Model file for the job. Use its own axes, mm. Face numbers are marked on the shaded views. Coordinates: 2 decimals unless noted, no trailing zeros. Write each loop counter-clockwise with the first axis right and the second up, starting at its lowest first coordinate (ties: lowest second). Pieces come first, ordered by that corner, then holes.
Q1. Band-saw the part on B-B, the plane z = 43. Write the cut outline in (x, y).
Q2. Drill centre lines: probe 1 along Z at (x, y) = (-50.5, -9); probe 2 along X at (y, z) = (-12, -38.5); probe 3 along X at (y, z) = (-3.5, 11.5). Where is each one in solid material? Low to high.
Q3. Band-saw the part on C-C, the plane y = -13. Write the cut outline in (x, z), plus the area to 3 significant figures.
Q4. Pin check, flat tip, straight feed: P1, Ø1.3, axis at y = -3.5, z = -17, coming from the -X side. Stop position of the tip, or through.
Q5. Band-saw the part on A-A, the plane x = -45. Write the cut outline in (y, z), plus the area to 3 significant figures.
Q6. Band-saw the part on D-D, the plane z = 19.5. Write the cut outline in (x, y).
Q7. Pull direction Z, two halves, no side cores. Call the marked faces 1, 2, 3 and 4: released by +Z, released by -Z, zero draft, split by the parting line, or undercut.
from build123d import *

# Parameters (mm, degrees)
F0_W      = 195.58
F0_H      = 127
F1_DEPTH  = 15.24
F2_W      = 2.54
F2_H      = 2.54
F3_DEPTH  = 127
F4_W      = 167.005
F4_H      = 70.993
F5_DEPTH  = 15.24
F6_W      = 172.085
F6_H      = 79.629
F7_DEPTH  = 11.43
F8_R      = 1.395268
F8_R_2    = 1.40268
F8_R_3    = 1.396073
F8_R_4    = 1.400056
F8_R_5    = 1.400396
F8_R_6    = 1.399702
F9_DEPTH  = 3.81
F10_W     = 193.04
F10_H     = 96.52
F11_DEPTH = 11.43


with BuildPart() as f1:
    # F0 (on Front) → F1 (new body)
    with BuildSketch(Plane.XZ):
        Rectangle(F0_W, F0_H)
    extrude(amount=F1_DEPTH)

    # F2 (on face) → F3 (cut)
    with BuildSketch(Plane.XY.offset(63.5)):
        with Locations((-96.52, -3.81)):
            Rectangle(F2_W, F2_H)
        with Locations((96.52, -3.81)):
            Rectangle(F2_W, F2_H)
    extrude(amount=-F3_DEPTH, mode=Mode.SUBTRACT)

    # F4 (on face) → F5 (cut)
    with BuildSketch(Plane.XZ.offset(15.24)):
        Rectangle(F4_W, F4_H)
    extrude(amount=-F5_DEPTH, mode=Mode.SUBTRACT)

    # F6 (on face) → F7 (cut)
    with BuildSketch(Plane.XZ.offset(15.24)):
        Rectangle(F6_W, F6_H)
    extrude(amount=-F7_DEPTH, mode=Mode.SUBTRACT)

    # F8 (on face) → F9 (cut)
    with BuildSketch(Plane.XZ.offset(3.81)):
        with Locations((0, 37.9857)):
            Circle(F8_R)
        with Locations((-83.5025, 37.9857)):
            Circle(F8_R_2)
        with Locations((-83.5025, -37.9857)):
            Circle(F8_R_3)
        with Locations((0, -37.9857)):
            Circle(F8_R_4)
        with Locations((83.5025, -37.9857)):
            Circle(F8_R_5)
        with Locations((83.5025, 37.9857)):
            Circle(F8_R_6)
    extrude(amount=-F9_DEPTH, mode=Mode.SUBTRACT)

    # F10 (on face) → F11 (cut)
    with BuildSketch(Plane.XZ.offset(15.24)):
        Rectangle(F10_W, F10_H)
    extrude(amount=-F11_DEPTH, mode=Mode.SUBTRACT)


solid = f1.part
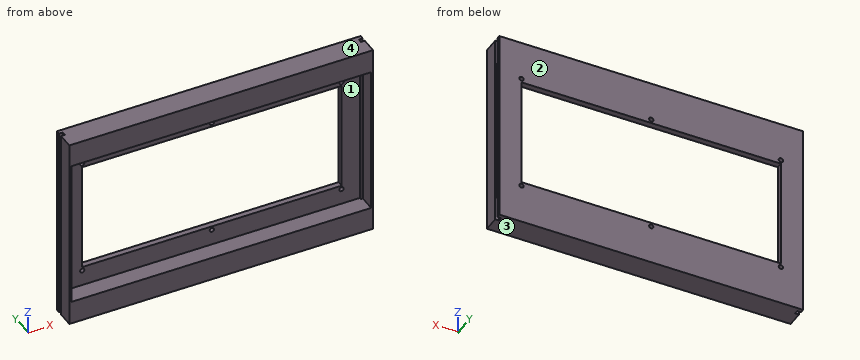
Answer sheet:
1. outline: (-97.79, -15.24) - (-96.52, -15.24) - (-96.52, -5.08) - (-97.79, -5.08) - close; (-97.79, -2.54) - (-95.25, -2.54) - (-95.25, -3.81) - (95.25, -3.81) - (95.25, -2.54) - (97.79, -2.54) - (97.79, 0) - (-97.79, 0) - close; (96.52, -15.24) - (97.79, -15.24) - (97.79, -5.08) - (96.52, -5.08) - close
2. probe 1: z = -63.5 to -48.26, 48.26 to 63.5
2. probe 2: x = -97.79 to -96.52, 96.52 to 97.79
2. probe 3: x = -95.25 to -83.5, 83.5 to 95.25
3. outline: (-97.79, -63.5) - (97.79, -63.5) - (97.79, 63.5) - (-97.79, 63.5) - close; hole (-96.52, -48.26) - (96.52, -48.26) - (96.52, 48.26) - (-96.52, 48.26) - close
3. area: 6,210 mm2
4. P1: stops at x = -95.25
5. outline: (-15.24, -63.5) - (0, -63.5) - (0, -35.5) - (-3.81, -35.5) - (-3.81, -48.26) - (-15.24, -48.26) - close; (-15.24, 48.26) - (-3.81, 48.26) - (-3.81, 35.5) - (0, 35.5) - (0, 63.5) - (-15.24, 63.5) - close
5. area: 562 mm2
6. outline: (-97.79, -15.24) - (-96.52, -15.24) - (-96.52, -5.08) - (-97.79, -5.08) - close; (-97.79, -2.54) - (-95.25, -2.54) - (-95.25, -3.81) - (-83.5, -3.81) - (-83.5, 0) - (-97.79, 0) - close; (83.5, -3.81) - (95.25, -3.81) - (95.25, -2.54) - (97.79, -2.54) - (97.79, 0) - (83.5, 0) - close; (96.52, -15.24) - (97.79, -15.24) - (97.79, -5.08) - (96.52, -5.08) - close
7. face 1: undercut
7. face 2: zero draft
7. face 3: released by -Z
7. face 4: released by +Z
